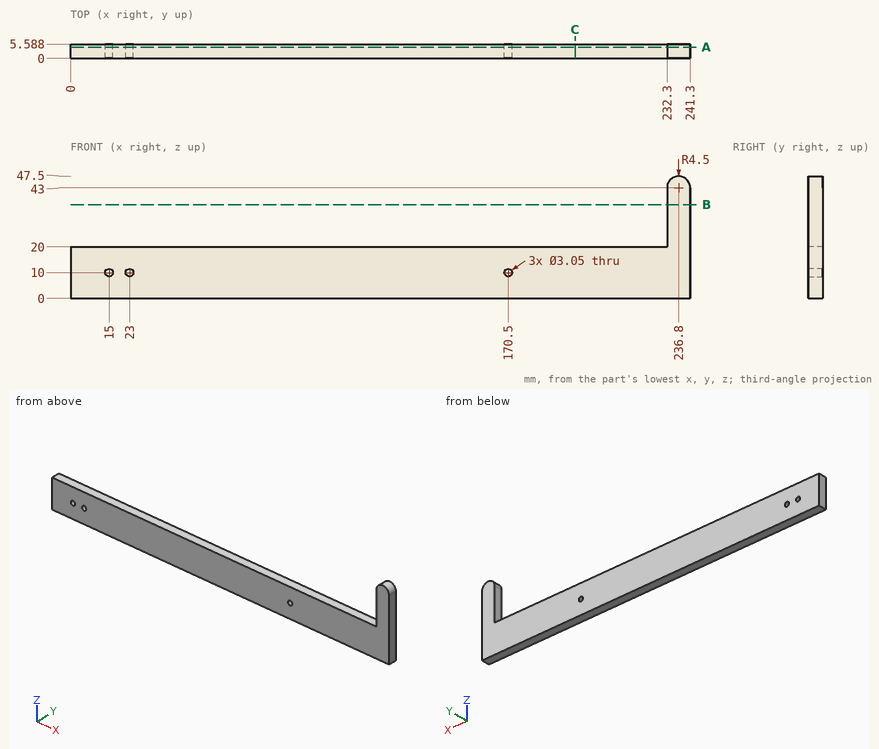
Part print with two shaded views. Sizes in mm from the minimum x, y, z corner. Round coordinates to 2 decimals unless told otherwise and drop trailing zeros. Write each loop counter-clockwise with the first axis right and the second up, starting at its lowest first coordinate (ties: lowest second). Pieces come first, ordered by that corner, then holes. Notation, with made-up numbers: M -4.75,52.25 L 42.25,52.25 A35 cw 42.25,90.25 Z; hole C 65,51.25 d11. An arc over 180 degrees is marked long. Put each result on its own line as item: value. Start each with the question number.
1) Pin check, flat tips, straight feed: pin 1 Ø3 at (x, y) = (63, 4) entering from +Z; pin 2 Ø4 at (x, z) = (23, 10) entering from +Y. Stop position of each tip, or through.
2) Drill centre lines: probe 1 along X at (y, z) = (2.45, 10) (3 decimals); probe 2 along Z at (x, y) = (15, 1.95) (3 decimals); probe 3 along Z at (x, y) = (188.5, 3.65). Where is each one in solid material? Low to high. Write a range as [from, to].
3) Saw through at C-C, the plane x = 196.5. Write the cut outline in (y, z), and give its area (3 significant figures).
4) Saw through at B-B, the plane z = 36.5. Write the cut outline in (x, y), and give its area (3 significant figures).
5) Saw through at A-A, the plane y = 4.35. Write the cut outline in (x, z) (3 decimals), and give its area (3 significant figures).
Resolved:
1. pin 1: z = 20
1. pin 2: y = 5.59
2. probe 1: [0, 13.475], [16.525, 21.475], [24.525, 168.975], [172.025, 241.3]
2. probe 2: [0, 8.475], [11.525, 20]
2. probe 3: [0, 20]
3. outline: M 0,0 L 5.59,0 L 5.59,20 L 0,20 Z
3. area: 112 mm²
4. outline: M 232.3,0 L 241.3,0 L 241.3,5.59 L 232.3,5.59 Z
4. area: 50.3 mm²
5. outline: M 0,0 L 241.3,0 L 241.3,43 A4.5 ccw 232.3,43 L 232.3,20 L 0,20 Z; hole C 15,10 d3.05; hole C 23,10 d3.05; hole C 170.5,10 d3.05
5. area: 5,040 mm²
